Can you work these out from the model? Positions are in its coordinate system, mm. A direction names the side the tool comes from. Give positions to 0.01 mm unless a question says otherwise; leave off trailing zeros. Order: outer loops, then holes, each group sorted by start corner. A loop starts at its lowest first (then second) coordinate and runs counter-clockwise, first axis right, second up. Notation, with made-up numbers: (61, 52) - (106, 52) arc R26 ccw to (106, 86) - close; hole circle Ø6 at (32.5, 60.25). An arc over 180 degrees is marked (long way). Use one line per item in the form item = value. Start each with the question number.
1) Suppose I cut it at B-B, the plane y = -5.75. Write out the boundary of the cut face in (x, z), and give its area (3 significant figures).
2) We'd pull the mould along Z, two halves only. Please class faces 1 (the flat face through (59, -7.5, 0)), 2 (the flat face through (59, 0, -12.5)), 3 (the cylindrical face through (4, 0, 0)): released by +Z, released by -Z, zero draft, split by the parting line, or undercut.
3) Please list where these lines run through material, in increasing order: probe 1 along Y at (x, z) = (100, 2.5); probe 2 along X at (y, z) = (-2.5, -10.5); probe 3 along X at (y, z) = (6, 6.5).
4) Suppose I cut it at A-A, the plane x = 115. Write out the boundary of the cut face in (y, z).
5) For pin 1 (10 mm diameter, centred on x = 14, z = 5, fed in from +Y); pin 2 (6.5 mm diameter, centred on y = 0.5, z = -8, fed in from +X); pin 3 (4.5 mm diameter, centred on y = -2.5, z = 8, fed in from +X), each with a flat end and sliding along its axis, tell me the tip position at first contact or that it passes through.
6) Which directions (+Z, -Z, +X, -X, +Y, -Y) give clear straight access to the entire face, cutting with the end or side of a thin tool? Please do faces 4 (the flat face through (120, 0, -11)), 5 (the flat face through (120, 0, 11)), 6 (the flat face through (0, 0, -8)).
7) Suppose I cut it at C-C, the plane z = -2. Write out the boundary of the cut face in (x, y).
```python
from build123d import *

# Parameters (mm, degrees)
SKETCH2_W           = 25
SKETCH2_H           = 15
BOSS_EXTRUDE1_DEPTH = 120
SKETCH3_R           = 4
CUT_EXTRUDE1_DEPTH  = 25


with BuildPart() as part:
    # Sketch2 → Boss-Extrude1 (new body)
    with BuildSketch(Plane(origin=(0, 0, 0), x_dir=(0, 0, -1), z_dir=(1, 0, 0))):
        Rectangle(SKETCH2_W, SKETCH2_H)
    extrude(amount=BOSS_EXTRUDE1_DEPTH)

    # Sketch3 → Cut-Extrude1 (cut)
    with BuildSketch(Plane(origin=(0, -12.5, 0), x_dir=(1, 0, 0), z_dir=(0, 1, 0))):
        Circle(SKETCH3_R)
    extrude(amount=CUT_EXTRUDE1_DEPTH, mode=Mode.SUBTRACT)

    # Sketch4 → Revolve1 (revolve)
    with BuildSketch(Plane.XY):
        with BuildLine():
            Line((120, -10), (120, 10))
            ThreePointArc((120, 10), (130, 0), (120, -10))
        make_face()
    revolve(axis=Axis((120, -10, 0), (0, 1, 0)))


solid = part.part
```
Result sheet:
q1.outline = (0, -12.5) - (120, -12.5) - (120, -8.18) arc R8.18 ccw to (120, 8.18) - (120, 12.5) - (0, 12.5) - (0, 4) arc R4 cw to (0, -4) - close
q1.area = 3,080 mm²
q2.face_1 = zero draft
q2.face_2 = released by -Z
q2.face_3 = undercut
q3.probe_1 = -7.5 to 7.5
q3.probe_2 = 0 to 120
q3.probe_3 = 0 to 124.66
q4.outline = (-7.5, -12.5) - (7.5, -12.5) - (7.5, -4.33) arc R8.66 ccw to (7.5, 4.33) - (7.5, 12.5) - (-7.5, 12.5) - (-7.5, 4.33) arc R8.66 ccw to (-7.5, -4.33) - close
q5.pin_1 = 7.5
q5.pin_2 = 128.79
q5.pin_3 = 127.9
q6.face_4 = -Z, +X
q6.face_5 = +Z, +X
q6.face_6 = +Z, -Z, -X, +Y, -Y
q7.outline = (3.46, -7.5) - (113.7, -7.5) arc R9.8 ccw (long way) to (113.7, 7.5) - (3.46, 7.5) - close
